from build123d import *

# Parameters (mm, degrees)
SK_ESTRIADO_R = 13.2
EJE_DEPTH     = 38.8


with BuildPart() as part:
    # Sk_Estriado → Eje (new body)
    with BuildSketch(Plane.XY.offset(2.5)):
        with BuildLine():
            Line((2.7, 17.189240821), (2.7, 16.17621711))
            ThreePointArc((2.7, 16.17621711), (0, 16.4), (-2.7, 16.17621711))
            Line((-2.7, 16.17621711), (-2.7, 17.189240821))
            ThreePointArc((-2.7, 17.189240821), (-6.328756096, 16.208233904), (-9.662140027, 14.47076536))
            Line((-9.662140027, 14.47076536), (-9.01524753, 13.699828903))
            ThreePointArc((-9.01524753, 13.699828903), (-10.541716799, 12.563128867), (-11.926216414, 11.257235986))
            Line((-11.926216414, 11.257235986), (-12.573108911, 12.028172443))
            ThreePointArc((-12.573108911, 12.028172443), (-15.068842026, 8.7), (-16.703257352, 4.874545499))
            Line((-16.703257352, 4.874545499), (-15.712160547, 4.699788392))
            ThreePointArc((-15.712160547, 4.699788392), (-16.150847149, 2.847830114), (-16.372023623, 0.957518931))
            Line((-16.372023623, 0.957518931), (-17.363120427, 1.132276038))
            ThreePointArc((-17.363120427, 1.132276038), (-17.135654902, -3.021478291), (-15.928734927, -7.002528375))
            Line((-15.928734927, -7.002528375), (-15.057179023, -6.49933534))
            ThreePointArc((-15.057179023, -6.49933534), (-14.202816622, -8.2), (-13.157179023, -9.790231874))
            Line((-13.157179023, -9.790231874), (-14.028734927, -10.293424909))
            ThreePointArc((-14.028734927, -10.293424909), (-11.184504409, -13.32917331), (-7.700980401, -15.603041398))
            Line((-7.700980401, -15.603041398), (-7.356776093, -14.657347834))
            ThreePointArc((-7.356776093, -14.657347834), (-5.609130351, -15.410958981), (-3.785944134, -15.957024379))
            Line((-3.785944134, -15.957024379), (-4.130148442, -16.902717943))
            ThreePointArc((-4.130148442, -16.902717943), (0, -17.4), (4.130148442, -16.902717943))
            Line((4.130148442, -16.902717943), (3.785944134, -15.957024379))
            ThreePointArc((3.785944134, -15.957024379), (5.609130351, -15.410958981), (7.356776093, -14.657347834))
            Line((7.356776093, -14.657347834), (7.700980401, -15.603041398))
            ThreePointArc((7.700980401, -15.603041398), (11.184504409, -13.32917331), (14.028734927, -10.293424909))
            Line((14.028734927, -10.293424909), (13.157179023, -9.790231874))
            ThreePointArc((13.157179023, -9.790231874), (14.202816622, -8.2), (15.057179023, -6.49933534))
            Line((15.057179023, -6.49933534), (15.928734927, -7.002528375))
            ThreePointArc((15.928734927, -7.002528375), (17.135654902, -3.021478291), (17.363120427, 1.132276038))
            Line((17.363120427, 1.132276038), (16.372023623, 0.957518931))
            ThreePointArc((16.372023623, 0.957518931), (16.150847149, 2.847830114), (15.712160547, 4.699788392))
            Line((15.712160547, 4.699788392), (16.703257352, 4.874545499))
            ThreePointArc((16.703257352, 4.874545499), (15.068842026, 8.7), (12.573108911, 12.028172443))
            Line((12.573108911, 12.028172443), (11.926216414, 11.257235986))
            ThreePointArc((11.926216414, 11.257235986), (10.541716799, 12.563128867), (9.01524753, 13.699828903))
            Line((9.01524753, 13.699828903), (9.662140027, 14.47076536))
            ThreePointArc((9.662140027, 14.47076536), (6.328756096, 16.208233904), (2.7, 17.189240821))
        make_face()
        Circle(SK_ESTRIADO_R, mode=Mode.SUBTRACT)
    extrude(amount=-EJE_DEPTH)


solid = part.part
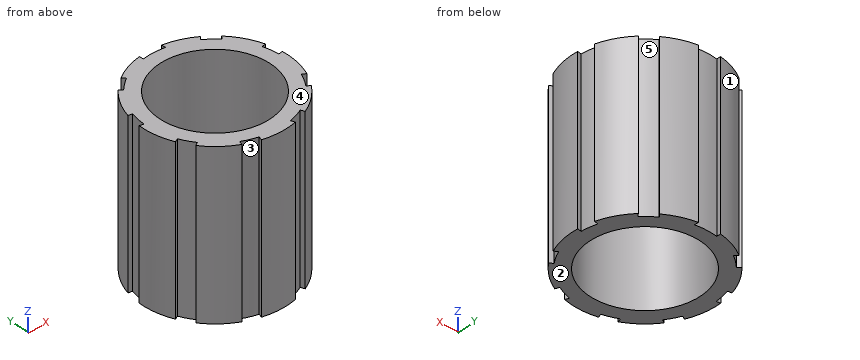
CAD build for the part. Positions are in the model's coordinates, mm. Face numbers are marked on the shaded views. A direction names the side the tool comes from. Give positions to 0.01 mm unless a question says otherwise; leave off trailing zeros. Loops run counter-clockwise (first coordinate to the right, second up) from the corner with the lowest first, then second, coordinate; pieces in that order, holes last. Notation, with made-up numbers: M 65,-40 L 121,-40 A29 ccw 121,-12 Z; hole C -38,-9 d4. An arc over 180 degrees is marked long. One line per question, with ' | ' between items. Start each with the question number.
1. Saw through at B-B on y = 0. Give the cut face in (x, z).
2. Saw through at A-A on x = 0. Give the cut face in (y, z), plus the area to 3 significant figures.
3. 3-axis set-ups, long thin cutter, end or side, ignore diameter. For the marked faces 4 and 5: which of +Z, -Z, +X, -X, +Y, -Y reach the whole face in a straight line?
4. Two-plate mould, pull along X, no slides. Class the marked faces 1, 2 and 3: pulls with the +X half, pulls with the -X half, needs draft (parallel to the pull), parting line crosses it, or undercut.
5. Flat gauge pins, fed straight in: pin 1 (2 mm diameter, centred on x = -12.5, y = 13.5, fed in from +Z); pin 2 (4 mm diameter, centred on x = 5, z = -15.5, fed in from -Y); pin 3 (12 mm diameter, centred on y = 8, z = -17.5, fed in from +X); pin 4 (10 mm diameter, centred on x = 8, y = -7, fed in from -Z). Where does each tip first touch, or does it go through?
6. Probe L1, parallel to Y at x = 0, z = -13; L2, parallel to X at y = -1, z = -8; L3, parallel to X at y = -5.5, z = -24. List the from-to ranges inside material, lowest first. Write a range as from..to.
Result sheet:
1) outline: M -17.4,-36.3 L -13.2,-36.3 L -13.2,2.5 L -17.4,2.5 Z; M 13.2,-36.3 L 17.4,-36.3 L 17.4,2.5 L 13.2,2.5 Z
2) outline: M -17.4,-36.3 L -13.2,-36.3 L -13.2,2.5 L -17.4,2.5 Z; M 13.2,-36.3 L 16.4,-36.3 L 16.4,2.5 L 13.2,2.5 Z | area: 287 mm^2
3) face 4: +Z, +X, -X, +Y, -Y | face 5: +Z, -Z
4) face 1: pulls with the -X half | face 2: needs draft | face 3: undercut
5) pin 1: passes through | pin 2: stops at y = -17.14 | pin 3: stops at x = 16.7 | pin 4: stops at z = -36.3
6) L1: y = -17.4..-13.2, 13.2..16.4 | L2: x = -17.37..-13.16, 13.16..17.37 | L3: x = -16.51..-12, 12..16.51
